Geometry check sheet. Reference: the model listing, model coordinates, mm. Face numbers are marked on the shaded views. Round coordinates to 2 decimals unless told otherwise and drop trailing zeros. Write each loop counter-clockwise with the first axis right and the second up, starting at its lowest first coordinate (ties: lowest second). Pieces come first, ordered by that corner, then holes. Notation, with made-up numbers: M -10.5,43 L 9.5,43 A34 ccw 9.5,82 Z; hole C -32.5,15 d4. An arc over 180 degrees is marked long. Use a Markdown table: item, result.
Autodesk Inventor part; units mm, degrees
ref_plane "YZ Plane" through (0, 0, 0) normal (1, 0, 0) x (0, 1, 0)
ref_plane "XZ Plane" through (0, 0, 0) normal (0, 1, 0) x (-1, 0, 0)
ref_plane "XY Plane" through (0, 0, 0) normal (0, 0, 1) x (1, 0, 0)
sketch "スケッチ1" plane through (0, 0, 0) normal (0, 1, 0) x (-1, 0, 0)
  circle A0 centre (0, 0) radius 45
  circle A1 centre (0, 0) radius 57.5
  dimension "d0" = 90
  dimension "d1" = 115
extrude "押し出し1" add sketch "スケッチ1" along normal blind 8.5
sketch "スケッチ2" plane through (0, 8.5, 0) normal (0, 1, 0) x (1, 0, 0)
  point P0 (0, 0)
  point P1 (-50.5, 0)
  point P2 (0, -50.5)
  point P3 (50.5, 0)
  point P4 (0, 50.5)
  dimension "d4" = 50.5
  dimension "d7" = 360
hole "穴1" at (-50.5, 8.5, 0) at (0, 8.5, 50.5) at (50.5, 8.5, 0) at (0, 8.5, -50.5) direction (0, -1, 0) diameter 5 end through all
properties part number "turntable1" material "アルミニウム 6061"
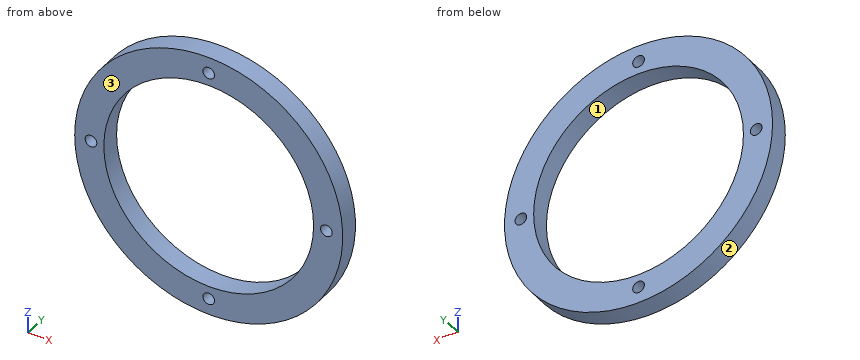
Item 1: Cross-section at A-A, the plane x = 0. Record the cut outline in (y, z).
Outcome:
| item | result |
|---|---|
| outline | M 0,-57.5 L 8.5,-57.5 L 8.5,-53 L 0,-53 Z; M 0,-48 L 8.5,-48 L 8.5,-45 L 0,-45 Z; M 0,45 L 8.5,45 L 8.5,48 L 0,48 Z; M 0,53 L 8.5,53 L 8.5,57.5 L 0,57.5 Z |
Item 2: Cross-section at B-B, the plane z = 0. Record the cut outline in (x, y), and give its area (4 significant figures).
Outcome:
| item | result |
|---|---|
| outline | M -57.5,0 L -53,0 L -53,8.5 L -57.5,8.5 Z; M -48,0 L -45,0 L -45,8.5 L -48,8.5 Z; M 45,0 L 48,0 L 48,8.5 L 45,8.5 Z; M 53,0 L 57.5,0 L 57.5,8.5 L 53,8.5 Z |
| area | 127.5 mm2 |
Item 3: Go/stop test with flat-tipped pins: pin 1 (1 mm diameter, centred on x = -0.5, y = 1.5, fed in from -Z); pin 2 (4 mm diameter, centred on x = 22, y = 4, fed in from -Z); pin 3 (3 mm diameter, centred on x = -50.5, z = 0, fed in from -Y); pin 4 (5 mm diameter, centred on y = 4, z = -14.5, fed in from -X). Record where each tip stops, or that it passes through.
Outcome:
| item | result |
|---|---|
| pin 1 | stops at z = -57.5 |
| pin 2 | stops at z = -53.91 |
| pin 3 | passes through |
| pin 4 | stops at x = -56.23 |
Item 4: Material ranges on line 1 along Z through (x, y) = (0, 5); line 2 along X through (y, z) = (4.5, 16); line 3 along X through (y, z) = (2.5, -50.5), recorded low to high. Write a range as from..to.
Outcome:
| item | result |
|---|---|
| line 1 | z = -57.5..-53, -48..-45, 45..48, 53..57.5 |
| line 2 | x = -55.23..-42.06, 42.06..55.23 |
| line 3 | x = -27.5..-2.5, 2.5..27.5 |
Item 5: Mould release check, pull along X, two halves, no side actions. Record for the marked faces 1, 2 and 3: +X half, -X half, draft (parallel to the pull), parting line (faces both ways), or undercut.
Outcome:
| item | result |
|---|---|
| face 1 | undercut |
| face 2 | parting line |
| face 3 | draft |
Item 6: Cross-section at C-C, the plane x = -36. Record the cut outline in (y, z), and give its area (3 significant figures).
Outcome:
| item | result |
|---|---|
| outline | M 0,-44.84 L 8.5,-44.84 L 8.5,-27 L 0,-27 Z; M 0,27 L 8.5,27 L 8.5,44.84 L 0,44.84 Z |
| area | 303 mm2 |
Item 7: Cross-section at D-D, the plane y = 5.5. Record the cut outline in (x, z).
Outcome:
| item | result |
|---|---|
| outline | C 0,0 d115; hole C -50.5,0 d5; hole C 0,0 d90; hole C 0,-50.5 d5; hole C 0,50.5 d5; hole C 50.5,0 d5 |
